The figure shows three views and two pictorial views of one solid part (mm, origin at its lowest corner). Answer the questions. A direction names the side the tool comes from. Give positions to 0.01 mm unless a question says otherwise; leave off trailing zeros. Write each loop counter-clockwise with the first axis right and the second up, starting at its lowest first coordinate (ties: lowest second). Pieces come first, ordered by that corner, then holes. Notation, with made-up numbers: (-14, 22.25) -> (39, 22.25) arc R24 cw to (39, 52.25) -> close; hole circle Ø2 at (72.5, 57). An arc over 180 degrees is marked (long way). Use a Markdown table: item, result.
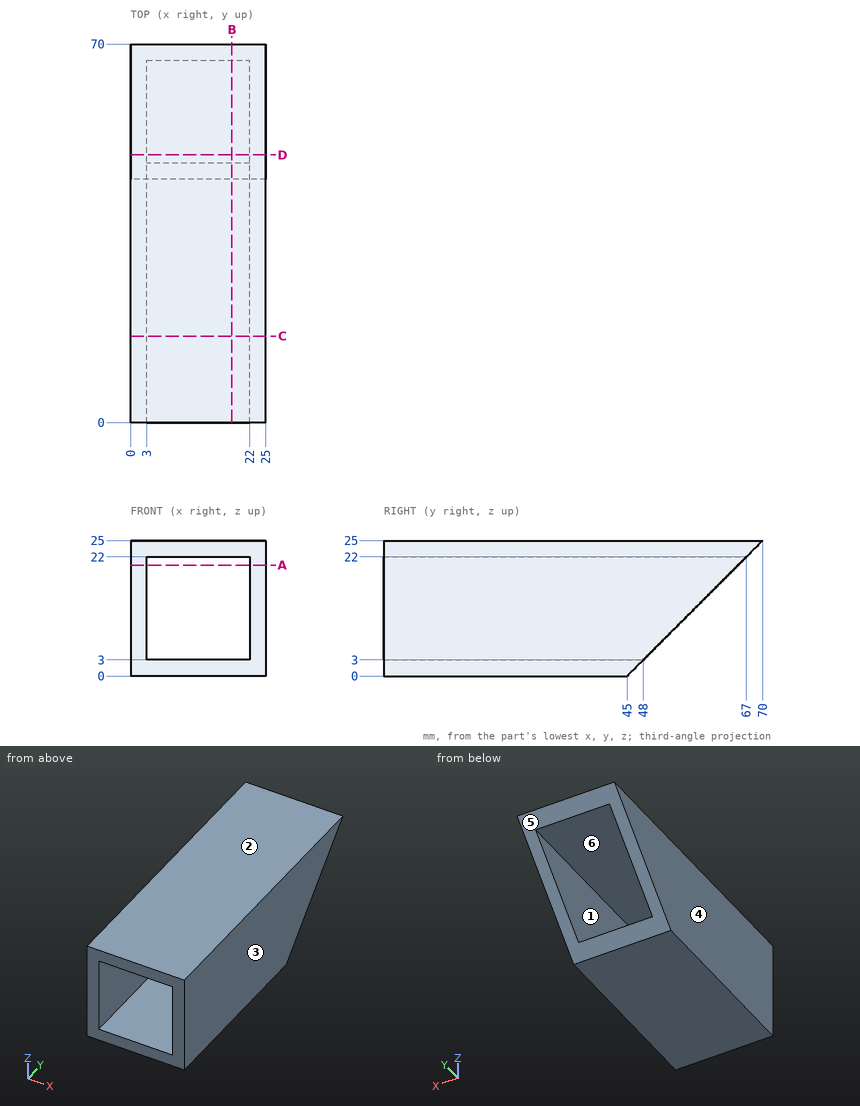
Item 1: Straight lines are drawn through the part: line 1 along X through (y, z) = (20, 16.75); line 2 along Z through (x, y) = (8.5, 51). For each, find the intervals that lie inside material, in ascending order. Write a range as [from, to].
Return value:
| item | result |
|---|---|
| line 1 | [0, 3], [22, 25] |
| line 2 | [22, 25] |
Item 2: A cutting plane is placed at D-D (y = 49.5). Give the vertices of the cut face in (x, z), then the cut area to 3 significant figures.
Return value:
| item | result |
|---|---|
| outline | (0, 4.5) -> (3, 4.5) -> (3, 22) -> (22, 22) -> (22, 4.5) -> (25, 4.5) -> (25, 25) -> (0, 25) -> close |
| area | 180 mm^2 |
Item 3: For a pull along X with two mould halves and no side action, classify the marked faces 3, 4, 5 and 6 as +X half, -X half, draft (parallel to the pull), parting line (faces both ways), or undercut.
Return value:
| item | result |
|---|---|
| face 3 | +X half |
| face 4 | -X half |
| face 5 | draft |
| face 6 | undercut |
Item 4: A cutting plane is placed at C-C (y = 16). Give the vertices of the cut face in (x, z).
Return value:
| item | result |
|---|---|
| outline | (0, 0) -> (25, 0) -> (25, 25) -> (0, 25) -> close; hole (3, 3) -> (22, 3) -> (22, 22) -> (3, 22) -> close |
Item 5: A tool of negligible diameter and unlimited length cuts with its end or side. For the marked faces 1 and 2, from which of +Z, -Z, +X, -X, +Y, -Y can it reach the whole face along a straight path? Write none if from no direction.
Return value:
| item | result |
|---|---|
| face 1 | +Y, -Y |
| face 2 | +Z, +X, -X, +Y, -Y |
Item 6: Each of these flat-tipped pins is pushed along its axis until it touches: P1, Ø2, axis at x = 20, z = 6.5, coming from the +Y side; P2, Ø4, axis at x = 4.5, z = 13, coming from the +Y side; P3, Ø8, axis at x = 21.5, z = 3.5, coming from the -Y side. Where does it stop, or does it pass through?
Return value:
| item | result |
|---|---|
| P1 | through |
| P2 | y = 59.32 |
| P3 | y = 0 |
Item 7: A cutting plane is placed at A-A (z = 20.5). Give the vertices of the cut face in (x, y), then the cut area to 3 significant figures.
Return value:
| item | result |
|---|---|
| outline | (0, 0) -> (3, 0) -> (3, 65.5) -> (0, 65.5) -> close; (22, 0) -> (25, 0) -> (25, 65.5) -> (22, 65.5) -> close |
| area | 393 mm^2 |
Item 8: A cutting plane is placed at B-B (x = 18.75). Give the vertices of the cut face in (y, z), then the cut area to 3 significant figures.
Return value:
| item | result |
|---|---|
| outline | (0, 0) -> (45, 0) -> (48, 3) -> (0, 3) -> close; (0, 22) -> (67, 22) -> (70, 25) -> (0, 25) -> close |
| area | 345 mm^2 |
